Could you check a few things on this model? Use its own coordinates, in mm. Coordinates: 2 decimals unless noted, no trailing zeros. Order: outer loops, then holes, each group sorted by start corner. A loop starts at its lowest first (then second) coordinate and runs counter-clockwise, first axis right, second up. Notation, with made-up numbers: (75, 5.5) - (103, 5.5) arc R13 ccw to (103, 24.5) - close; hole circle Ø2 at (-22.5, -22). An arc over 180 degrees is marked (long way). Answer as a JSON object with one key per item and string values. Group by question number.
(1) Imagine slicing it at A-A, the plane z = -18.5. Write out the boundary of the cut face in (x, y).
(2) Imagine slicing it at C-C, the plane y = 2. Give the number of separate pieces and of enclosed holes in the cut face, and give its area (3 significant figures).
(3) Please list where these lines run through material, in increasing order: probe 1 along Z at (x, y) = (62.5, 2.4); probe 2 along Z at (x, y) = (-20.5, 2.6); probe 3 along Z at (x, y) = (-62, 1).
(4) Will these pins go through, and if not, where does the flat tip stop? P1, Ø1.5, axis at y = 1, z = -127, coming from the -X side; P2, Ø3.5, axis at x = -47.5, z = -55, coming from the +Y side (3 decimals); P3, Ø1, axis at x = 4, y = 0.5, coming from the +Z side; P4, Ø1.5, axis at x = 51.5, y = 1.5, coming from the -Z side.
(5) Imagine slicing it at B-B, the plane x = 26.5. Write out the boundary of the cut face in (y, z).
from build123d import *

# Parameters (mm, degrees)
SKETCH_1_R          = 2
EXTRUDE_1_DEPTH     = 3
SKETCH_3_W          = 80
SKETCH_3_H          = 109
CUT_EXTRUDE_2_DEPTH = 147.799182559
SKETCH_2_R          = 1
CUT_EXTRUDE_1_DEPTH = 147.799182559
SKETCH_5_W          = 6
SKETCH_5_H          = 54.5
EXTRUDE_1_2_DEPTH   = 3
FILLET_1_R          = 2
FILLET_2_R          = 1
FILLET_3_R          = 3


with BuildPart() as part:
    # 草图1 → Extrude 1 (new body)
    with BuildSketch(Plane(origin=(0, 0, 0), x_dir=(1, 0, 0), z_dir=(0, 1, 0))):
        Polygon((-17.5, 0), (17.5, 0), (17.5, -3), (47.5, -3), (47.5, 0), (70, 0), (70, 125), (40, 125), (40, 129), (15, 129), (15, 125), (-15, 125), (-15, 129), (-40, 129), (-40, 125), (-70, 125), (-70, 0), (-47.5, 0), (-47.5, -3), (-17.5, -3), align=None)
        with Locations(Location((47.5, 80, 0), (0, 0, 270))):
            Circle(SKETCH_1_R, mode=Mode.SUBTRACT)
        with Locations(Location((47.5, 55, 0), (0, 0, 270))):
            Circle(SKETCH_1_R, mode=Mode.SUBTRACT)
        with Locations(Location((-47.5, 55, 0), (0, 0, 90))):
            Circle(SKETCH_1_R, mode=Mode.SUBTRACT)
        with Locations(Location((-47.5, 80, 0), (0, 0, 90))):
            Circle(SKETCH_1_R, mode=Mode.SUBTRACT)
        with Locations(Location((-62.5, 30, 0), (0, 0, 270))):
            Circle(SKETCH_1_R, mode=Mode.SUBTRACT)
        with Locations(Location((-62.5, 62.5, 0), (0, 0, 270))):
            Circle(SKETCH_1_R, mode=Mode.SUBTRACT)
        with Locations(Location((-62.5, 95, 0), (0, 0, 270))):
            Circle(SKETCH_1_R, mode=Mode.SUBTRACT)
        with Locations(Location((62.5, 95, 0), (0, 0, 90))):
            Circle(SKETCH_1_R, mode=Mode.SUBTRACT)
        with Locations(Location((62.5, 62.5, 0), (0, 0, 90))):
            Circle(SKETCH_1_R, mode=Mode.SUBTRACT)
        with Locations(Location((62.5, 30, 0), (0, 0, 90))):
            Circle(SKETCH_1_R, mode=Mode.SUBTRACT)
    extrude(amount=EXTRUDE_1_DEPTH)

    # 草图3 → 切除-拉伸2 (cut, through all)
    with BuildSketch(Plane(origin=(0, 3, 0), x_dir=(1, 0, 0), z_dir=(0, 1, 0))):
        Polygon((-60, 117), (-46, 90), (-46, 117), align=None)
        Polygon((46, 8), (46, 42.5), (60, 8), align=None)
        with Locations((0, 62.5)):
            Rectangle(SKETCH_3_W, SKETCH_3_H)
        Polygon((-46, 42.5), (-60, 8), (-46, 8), align=None)
        Polygon((46, 117), (60, 117), (46, 90), align=None)
    extrude(amount=-CUT_EXTRUDE_2_DEPTH, mode=Mode.SUBTRACT)

    # 草图2 → 切除-拉伸1 (cut, through all)
    with BuildSketch(Plane(origin=(0, 3, 0), x_dir=(1, 0, 0), z_dir=(0, 1, 0))):
        with Locations((-48.5, 0)):
            Circle(SKETCH_2_R)
        with Locations((-16.5, 0)):
            Circle(SKETCH_2_R)
        with Locations((16.5, 0)):
            Circle(SKETCH_2_R)
        with Locations((14, 125)):
            Circle(SKETCH_2_R)
        with Locations((-41, 125)):
            Circle(SKETCH_2_R)
        with Locations((-14, 125)):
            Circle(SKETCH_2_R)
        with Locations((41, 125)):
            Circle(SKETCH_2_R)
        with Locations((48.5, 0)):
            Circle(SKETCH_2_R)
    extrude(amount=-CUT_EXTRUDE_1_DEPTH, mode=Mode.SUBTRACT)

    # 草图5 → Extrude 1 2 (add)
    with BuildSketch(Plane(origin=(0, 3, 0), x_dir=(1, 0, 0), z_dir=(0, 1, 0))):
        Polygon((-41.689048685, 114.52066248), (34.67155679, 62.5), (-41.689048685, 10.47933752), (-38.310951315, 5.52066248), (45.32844321, 62.5), (-38.310951315, 119.47933752), align=None)
        Polygon((41.689048685, 10.47933752), (-34.67155679, 62.5), (41.689048685, 114.52066248), (38.310951315, 119.47933752), (-45.32844321, 62.5), (38.310951315, 5.52066248), align=None)
        with Locations((0, 62.5)):
            Rectangle(SKETCH_5_W, SKETCH_5_H)
    extrude(amount=-EXTRUDE_1_2_DEPTH)

    # 圆角1
    fillet_1_edges = [part.edges().sort_by_distance(p)[0] for p in [
        (46, 1.5, -90),
        (46, 1.5, -117),
        (60, 1.5, -117),
        (60, 1.5, -8),
        (46, 1.5, -8),
        (46, 1.5, -42.5),
        (-46, 1.5, -42.5),
        (-46, 1.5, -8),
        (-60, 1.5, -8),
        (-60, 1.5, -117),
        (-46, 1.5, -117),
        (-46, 1.5, -90),
        (34.67155679, 1.5, -8),
        (-34.67155679, 1.5, -8),
        (40, 1.5, -11.630001937),
        (40, 1.5, -113.369998063),
        (40, 1.5, -66.130001937),
        (40, 1.5, -58.869998063),
        (34.67155679, 1.5, -117),
        (-34.67155679, 1.5, -117),
        (-40, 1.5, -11.630001937),
        (-40, 1.5, -113.369998063),
        (-40, 1.5, -58.869998063),
        (-40, 1.5, -66.130001937),
        (-5.32844321, 1.5, -89.75),
        (-5.32844321, 1.5, -35.25),
        (0, 1.5, -93.380001937),
        (5.32844321, 1.5, -35.25),
        (5.32844321, 1.5, -89.75),
        (0, 1.5, -31.619998063),
        (3, 1.5, -84.076248063),
        (34.67155679, 1.5, -62.5),
        (3, 1.5, -40.923751937),
        (-34.67155679, 1.5, -62.5),
        (-3, 1.5, -40.923751937),
        (-3, 1.5, -84.076248063),
    ]]
    fillet(fillet_1_edges, radius=FILLET_1_R)

    # 圆角2
    fillet_2_edges = [part.edges().sort_by_distance(p)[0] for p in [
        (47.5, 1.5, 3),
        (17.5, 1.5, 3),
        (-17.5, 1.5, 3),
        (-47.5, 1.5, 3),
        (-40, 1.5, -129),
        (-15, 1.5, -129),
        (15, 1.5, -129),
        (40, 1.5, -129),
    ]]
    fillet(fillet_2_edges, radius=FILLET_2_R)

    # 圆角3
    fillet_3_edges = [part.edges().sort_by_distance(p)[0] for p in [
        (70, 1.5, -125),
        (70, 1.5, 0),
        (-70, 1.5, 0),
        (-70, 1.5, -125),
    ]]
    fillet(fillet_3_edges, radius=FILLET_3_R)


solid = part.part
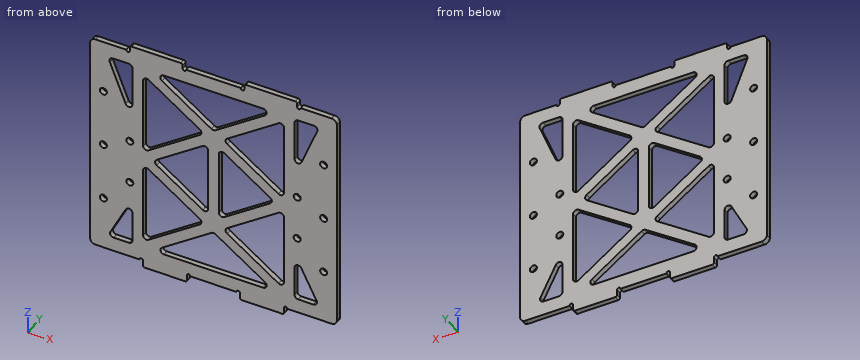
Result set:
{
 "1": {"outline": "(-70, 0) - (-55.74, 0) - (-55.74, 3) - (-70, 3) - close; (-46, 0) - (-40, 0) - (-40, 3) - (-46, 3) - close; (-29.92, 0) - (-19.26, 0) - (-19.26, 3) - (-29.92, 3) - close; (19.26, 0) - (29.92, 0) - (29.92, 3) - (19.26, 3) - close; (40, 0) - (46, 0) - (46, 3) - (40, 3) - close; (55.74, 0) - (70, 0) - (70, 3) - (55.74, 3) - close"},
 "2": {"separate pieces": "1", "enclosed holes": "22", "area": "10,700 mm^2"},
 "3": {"probe 1": "z = -125 to -97, -93 to -64.5, -60.5 to -32, -28 to 0", "probe 2": "z = -129 to -117, -107.35 to -100.09, -79.41 to -72.15, -52.85 to -45.59, -24.91 to -17.65, -8 to 3", "probe 3": "z = -125 to -96.94, -93.06 to -64.44, -60.56 to -31.94, -28.06 to 0"},
 "4": {"P1": "stops at x = -40", "P2": "passes through", "P3": "stops at z = 0", "P4": "stops at z = -125"},
 "5": {"outline": "(0, -129) - (3, -129) - (3, -117) - (0, -117) - close; (0, -111.43) - (3, -111.43) - (3, -104.17) - (0, -104.17) - close; (0, -75.33) - (3, -75.33) - (3, -68.07) - (0, -68.07) - close; (0, -56.93) - (3, -56.93) - (3, -49.67) - (0, -49.67) - close; (0, -20.83) - (3, -20.83) - (3, -13.57) - (0, -13.57) - close; (0, -8) - (3, -8) - (3, 3) - (0, 3) - close"}
}
